Input: part model. Units: mm. Frame: model coordinates. A direction names the side the tool comes from. Round coordinates to 2 decimals unless told otherwise and drop trailing zeros. Write each loop counter-clockwise with the first axis right and the second up, starting at its lowest first coordinate (ties: lowest second). Pieces come first, ordered by that corner, then holes. Notation, with made-up numbers: (52.25, 53) -> (106.25, 53) arc R12 ccw to (106.25, 64) -> close; hole circle Ø4 at (20, -26). An arc over 180 degrees is marked (long way). Write item = value, one per line.
```python
from build123d import *

# Parameters (mm, degrees)
EXTRUDE_1_DEPTH     = 16
SKETCH_3_R          = 1.5
CUT_EXTRUDE_1_DEPTH = 82.804645345
SKETCH_4_W          = 6
SKETCH_4_H          = 6
EXTRUDE_2_DEPTH     = 16
EXTRUDE_START       = -16
EXTRUDE_4_DEPTH     = 8


with BuildPart() as part:
    # Эскиз1 → Бобышка-Вытянуть1 (new body)
    with BuildSketch(Plane(origin=(0, 0, 0), x_dir=(1, 0, 0), z_dir=(0, 1, 0))):
        Polygon((0, 0), (-71.525936721, 0), (-71.525936721, 1.396480231), (-71.325936721, 1.396480231), (-71.325936721, 2.8586364), (-75.035652424, 2.8586364), (-80, -0.007531009), (-80, -6), (70, -6), (70, 0), align=None)
    extrude(amount=EXTRUDE_1_DEPTH)

    # Эскиз3 → Вырез-Вытянуть1 (cut, through all)
    with BuildSketch(Plane(origin=(0, 16, 0), x_dir=(1, 0, 0), z_dir=(0, 1, 0))):
        with Locations(Location((8.699103215, -3.003765504, 0), (0, 0, 270))):
            Circle(SKETCH_3_R)
        with Locations(Location((58.699103215, -3.003765504, 0), (0, 0, 270))):
            Circle(SKETCH_3_R)
        Polygon((-47.243192472, 0), (-45.239426968, -2.003765504), (-20.270391363, -2.003765504), (-18.266625858, 0), align=None)
        Polygon((-47.243192472, -6.007531009), (-18.266625858, -6.007531009), (-20.270391363, -4.003765504), (-45.239426968, -4.003765504), align=None)
    extrude(amount=-CUT_EXTRUDE_1_DEPTH, mode=Mode.SUBTRACT)

    # Эскиз4 → Бобышка-Вытянуть2 (add)
    with BuildSketch(Plane.XZ):
        with Locations((-69, 9)):
            Rectangle(SKETCH_4_W, SKETCH_4_H)
    extrude(amount=-EXTRUDE_2_DEPTH)

    # Эскиз5<2> → Бобышка-Вытянуть4 (add)
    with BuildSketch(Plane(origin=(0, 16, 0), x_dir=(1, 0, 0), z_dir=(0, 1, 0)).offset(EXTRUDE_START)):
        Polygon((-72, -12), (-72, -6), (-66, -9), (-66, -12), align=None)
    extrude(amount=-EXTRUDE_4_DEPTH)


solid = part.part
```
1) First-contact query: P1, Ø3, axis at x = 3, y = -1, coming from the +Z side; P2, Ø3, axis at y = 8, z = 10, coming from the -X side; P3, Ø3, axis at y = -2, z = 7, coming from the +X side. Flat tips, straight axial feed; report the tip coordinate or a pass-through.
Solutions:
P1 = 6
P2 = -72
P3 = -67
2) Cut plane C-C (y = -5.75). Return the cut outline in (x, z), and give its area (3 significant figures).
Solutions:
outline = (-72, 6) -> (-66, 9) -> (-66, 12) -> (-72, 12) -> close
area = 27.0 mm^2
3) Line query: L1, parallel to Z at x = 9, y = 6.25; L2, parallel to X at y = 6.5, z = 6.75; L3, parallel to Y at x = -23.5, z = 3.5. Output: solid intervals per line, ascending. Write a range as from..to.
Solutions:
L1 = 0..1.53, 4.47..6
L2 = -72..-66
L3 = 0..16
4) Access query for faces 4 (the face through (26, 8, 0)), 5 (the face through (-33, 8, 2.004)), 6 (the face through (-66, 7, 9)). Directions: +Z, -Z, +X, -X, +Y, -Y. A direction counts if a zero-diameter tool reaches every point of the face in a straight line with its end or side. Return the directions, or none.
Solutions:
face_4 = -Z, +X, +Y, -Y
face_5 = -Z, +Y, -Y
face_6 = +Z, +X, +Y, -Y
5) Cut plane A-A (y = 13.5). Return the cut outline in (x, z).
Solutions:
outline = (-80, 0.01) -> (-75.04, -2.86) -> (-71.33, -2.86) -> (-71.33, -1.4) -> (-71.53, -1.4) -> (-71.53, 0) -> (-47.24, 0) -> (-45.24, 2) -> (-20.27, 2) -> (-18.27, 0) -> (70, 0) -> (70, 6) -> (-18.27, 6) -> (-20.27, 4) -> (-45.24, 4) -> (-47.24, 6) -> (-66, 6) -> (-66, 12) -> (-72, 12) -> (-72, 6) -> (-80, 6) -> close; hole circle Ø3 at (8.7, 3); hole circle Ø3 at (58.7, 3)
6) Cut plane B-B (x = -44). Return the cut outline in (y, z), and give its area (3 significant figures).
Solutions:
outline = (0, 2) -> (16, 2) -> (16, 4) -> (0, 4) -> close
area = 32.0 mm^2
7) Draft query along Z for faces 1 (the face through (-57, 8, 6)), 2 (the face through (-72, 4, 9)), 3 (the face through (60.186, 8.112, 2.808)). Return one class per face: +Z half, -Z half, draft (parallel to the pull), parting line (faces both ways), or undercut.
Solutions:
face_1 = +Z half
face_2 = draft
face_3 = undercut
